Job drawing, mm, ordinate dimensions from the low corner. One solid piece. Give positions to 0.01 mm unless a question says otherwise; leave off trailing zeros. Write each loop counter-clockwise with the first axis right and the second up, starting at its lowest first coordinate (ties: lowest second). Pieces come first, ordered by that corner, then holes. Notation, with made-up numbers: (-17.75, -27) -> (33.25, -27) arc R23 ccw to (33.25, -16) -> close; hole circle Ø3 at (34, 38.25). An arc over 180 degrees is marked (long way). One line per question, with ' | ' between items. Start each with the question number.
(1) Pull direction Y, two halves, no side cores. Call the marked faces 1 and 2: released by +Y, released by -Y, zero draft, split by the parting line, or undercut.
(2) Band-saw the part on C-C, the plane z = 1. Give the cut face in (x, y).
(3) Drill centre lines: probe 1 along Y at (x, z) = (25, 0.8); probe 2 along Y at (x, z) = (26.5, 0.5); probe 3 along Y at (x, z) = (4, 1.15). Where is each one in solid material? Low to high. Write a range as from..to.
(4) Pin check, flat tips, straight feed: P1, Ø1.5, axis at x = 25.5, z = 2.5, coming from the +Y side; P2, Ø1.5, axis at y = 5.5, z = 2.5, coming from the -X side; P3, Ø4.5, axis at x = 25, y = 45, coming from the -Z side; P4, Ø1, axis at x = 33.5, z = 1, coming from the +Y side. Stop position of each tip, or through.
(5) Band-saw the part on A-A, the plane x = 25. Give the cut face in (y, z).
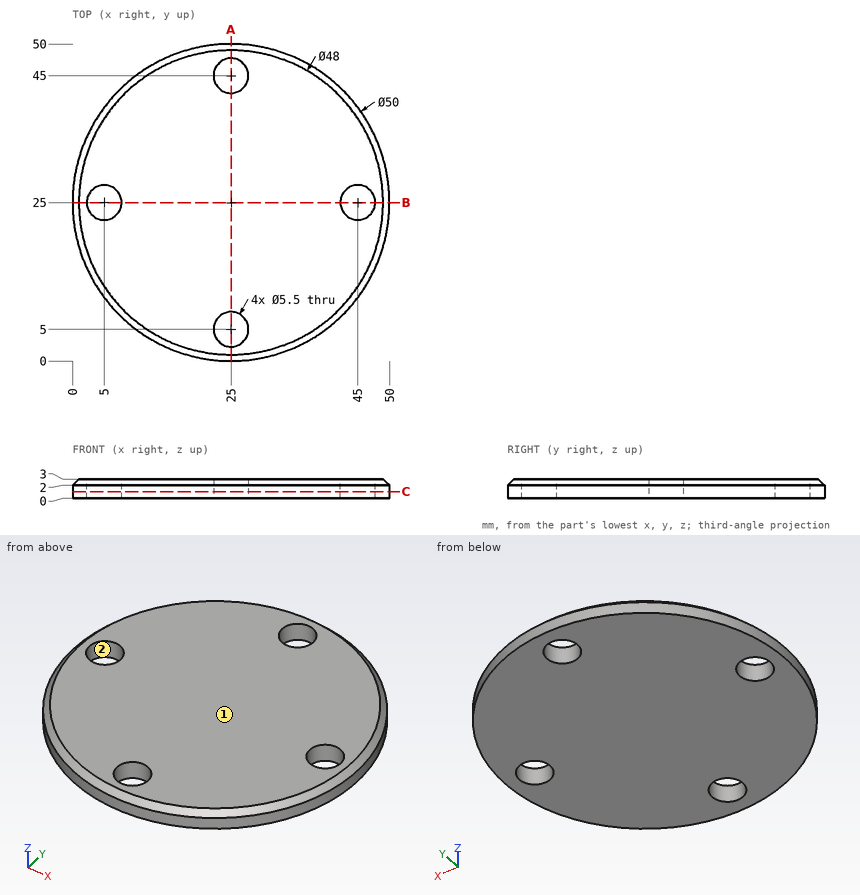
Results:
1) face 1: zero draft | face 2: undercut
2) outline: circle Ø50 at (25, 25); hole circle Ø5.5 at (5, 25); hole circle Ø5.5 at (25, 5); hole circle Ø5.5 at (25, 45); hole circle Ø5.5 at (45, 25)
3) probe 1: y = 0..2.25, 7.75..42.25, 47.75..50 | probe 2: y = 0.05..2.7, 7.3..42.7, 47.3..49.95 | probe 3: y = 11.44..22.44, 27.56..38.56
4) P1: stops at y = 50 | P2: stops at x = 8.68 | P3: passes through | P4: stops at y = 48.69
5) outline: (0, 0) -> (2.25, 0) -> (2.25, 3) -> (1, 3) -> (0, 2) -> close; (7.75, 0) -> (42.25, 0) -> (42.25, 3) -> (7.75, 3) -> close; (47.75, 0) -> (50, 0) -> (50, 2) -> (49, 3) -> (47.75, 3) -> close
